Verification items for the finished model (mm, model axes). A direction names the side the tool comes from. Round coordinates to 2 decimals unless told otherwise and drop trailing zeros. Write each loop counter-clockwise with the first axis right and the second up, starting at its lowest first coordinate (ties: lowest second). Pieces come first, ordered by that corner, then holes. Notation, with made-up numbers: M 2.5,81.5 L 54.5,81.5 A28 cw 54.5,118.5 Z; hole C 18.25,30.5 d2. An arc over 180 degrees is marked long. Answer in a Markdown table with one row per item. Add a question column.
1. Sectioned sample at A-A on y = 0. Record the cut outline in (x, z), plus the area to 3 significant figures.
2. Sectioned sample at B-B on z = 18.5. Record the cut outline in (x, y).
3. Sectioned sample at C-C on x = -4. Record the cut outline in (y, z).
4. Material ranges on probe 1 along Y at (x, z) = (0, 8.25); probe 2 along X at (y, z) = (5.5, 19); probe 3 along Y at (x, z) = (0, 17.5), recorded low to high.
5. Set-up check for faces 1 (the flat face through (-4, -11, 0)), 2 (the cylindrical face through (-5.19, -9.98, 6.9)): record each of +Z, -Z, +X, -X, +Y, -Y from which the full face is reachable in a straight line by a thin tool's end or side.
6. Draft check along Y on faces 3 (the flat face through (-7.605, -12.93, 10.55)), 4 (the flat face through (-2, 8, 14)), 5 (the flat face through (-3.5, -7.5, 21.4)). Enter one of: pulls with the +Y half, pulls with the -Y half, needs draft (parallel to the pull), parting line crosses it, or undercut.
7. Go/stop test with flat-tipped pins: pin 1 Ø13 at (x, y) = (0, 0) entering from +Z; pin 2 Ø1 at (x, y) = (5.5, 8.5) entering from -Z; pin 3 Ø1 at (x, z) = (9.5, 17.5) entering from +Y. Record where each tip stops, or that it passes through.
8. Sectioned sample at D-D on z = 9.5. Record the cut outline in (x, y).
```python
from build123d import *

# Parameters (mm, degrees)
BASE_EXTRUDE_DEPTH = 21.4
SKETCH2_R          = 11.25
CUT_EXTRUDE1_DEPTH = 14
SKETCH3_R          = 8
CUT_EXTRUDE2_DEPTH = 22.4


with BuildPart() as part:
    # Sketch1 → Base-Extrude (new body)
    with BuildSketch(Plane.XY):
        Polygon((0, 17.320508076), (-15, 8.660254038), (-15, -8.660254038), (0, -17.320508076), (15, -8.660254038), (15, 8.660254038), align=None)
    extrude(amount=BASE_EXTRUDE_DEPTH)

    # Sketch2 → Cut-Extrude1 (cut)
    with BuildSketch(Plane(origin=(0, 0, 0), x_dir=(-1, 0, 0), z_dir=(0, 0, -1))):
        Circle(SKETCH2_R)
    extrude(amount=-CUT_EXTRUDE1_DEPTH, mode=Mode.SUBTRACT)

    # Sketch3 → Cut-Extrude2 (cut, through all)
    with BuildSketch(Plane.XY.offset(21.4)):
        Circle(SKETCH3_R)
    extrude(amount=-CUT_EXTRUDE2_DEPTH, mode=Mode.SUBTRACT)


solid = part.part
```
Geometry check:
| question | item | result |
|---|---|---|
| 1 | outline | M -15,0 L -11.25,0 L -11.25,14 L -8,14 L -8,21.4 L -15,21.4 Z; M 8,14 L 11.25,14 L 11.25,0 L 15,0 L 15,21.4 L 8,21.4 Z |
| 1 | area | 209 mm2 |
| 2 | outline | M -15,-8.66 L 0,-17.32 L 15,-8.66 L 15,8.66 L 0,17.32 L -15,8.66 Z; hole C 0,0 d16 |
| 3 | outline | M -15.01,0 L -10.51,0 L -10.51,14 L -6.93,14 L -6.93,21.4 L -15.01,21.4 Z; M 6.93,14 L 10.51,14 L 10.51,0 L 15.01,0 L 15.01,21.4 L 6.93,21.4 Z |
| 4 | probe 1 | y = -17.32 to -11.25, 11.25 to 17.32 |
| 4 | probe 2 | x = -15 to -5.81, 5.81 to 15 |
| 4 | probe 3 | y = -17.32 to -8, 8 to 17.32 |
| 5 | face 1 | -Z, +X, -X, +Y, -Y |
| 5 | face 2 | -Z |
| 6 | face 3 | pulls with the -Y half |
| 6 | face 4 | undercut |
| 6 | face 5 | needs draft |
| 7 | pin 1 | passes through |
| 7 | pin 2 | stops at z = 14 |
| 7 | pin 3 | stops at y = 12.12 |
| 8 | outline | M -15,-8.66 L 0,-17.32 L 15,-8.66 L 15,8.66 L 0,17.32 L -15,8.66 Z; hole C 0,0 d22.5 |
